Geometry check sheet. Reference: drawing and pictorial views, mm from the part's lowest x, y, z. A direction names the side the tool comes from. Coordinates: 2 decimals unless noted, no trailing zeros. Loops run counter-clockwise (first coordinate to the right, second up) from the corner with the lowest first, then second, coordinate; pieces in that order, holes last. Notation, with made-up numbers: (33.5, 49) - (49.5, 49) arc R27 cw to (49.5, 83) - close; hole circle Ø4 at (-18.5, 55). An arc over 180 degrees is marked (long way). One line per item, written item: value.
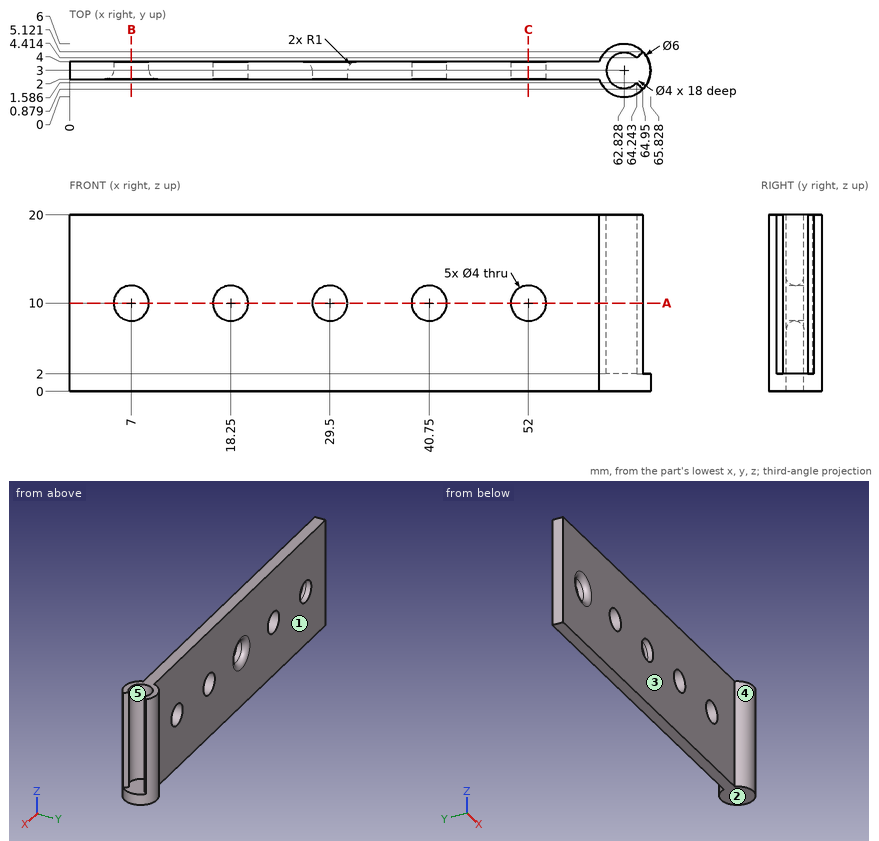
(1) Material ranges on probe 1 along Z at (x, y) = (29.5, 2.6); probe 2 along X at (y, z) = (2.3, 10.75) (1 decimal); probe 3 along Y at (x, z) = (14.5, 18.75), recorded low to high. Write a range as from..to.
Reply:
probe 1: 0..8, 12..20
probe 2: 0..4.8, 9.2..16.4, 20.1..27.6, 31.4..38.9, 42.6..50.1, 53.9..61
probe 3: 2..4
(2) Access from +Z, -Z, +X, -X, +Y, -Y to the whole of each face (thin tool, end or side, straight path). Record for the marked faces 1 and 2.
Reply:
face 1: +Z, -Z, -X, +Y
face 2: -Z, +X, -X, +Y, -Y
(3) Release check for a two-part mould opening along X. For the marked faces 3, 4 and 5 record: pulls with the +X half, pulls with the -X half, needs draft (parallel to the pull), parting line crosses it, or undercut.
Reply:
face 3: needs draft
face 4: parting line crosses it
face 5: undercut
(4) Go/stop test with flat-tipped pins: pin 1 Ø2 at (y, z) = (3.5, 8.5) entering from -X; pin 2 Ø8 at (x, z) = (10, 4) entering from +Y; pin 3 Ø6 at (x, z) = (16, 5) entering from -Y; pin 4 Ø1.3 at (x, y) = (62, 2) entering from +Z. Record where each tip stops, or that it passes through.
Reply:
pin 1: x = 0
pin 2: y = 4
pin 3: y = 2
pin 4: z = 2
(5) Cross-section at C-C on x = 52. Record the cut outline in (y, z).
Reply:
outline: (2, 0) - (4, 0) - (4, 8) - (2, 8) - close; (2, 12) - (4, 12) - (4, 20) - (2, 20) - close
(6) Cross-section at A-A on z = 10. State how many separate pieces and enclosed holes the cut face has.
Reply:
separate pieces: 6
enclosed holes: 0
(7) Cross-section at B-B on x = 7. Record the cut outline in (y, z).
Reply:
outline: (2, 0) - (4, 0) - (4, 8) - (3, 8) arc R1 ccw to (2, 7) - close; (2, 13) arc R1 ccw to (3, 12) - (4, 12) - (4, 20) - (2, 20) - close
